Read the model definition and answer for the solid it produces. Units are mm, in the model's axes. A direction names the side the tool comes from. Give positions to 0.01 mm unless a question says otherwise; leave off trailing zeros. Order: outer loops, then holes, each group sorted by start corner. A loop starts at its lowest first (then second) coordinate and runs counter-clockwise, first axis right, second up. Notation, with made-up numbers: (38, 80.5) - (93, 80.5) arc R20 ccw to (93, 107.5) - close; hole circle Ø8 at (-13.5, -37.5). An arc over 180 degrees is marked (long way). Write each question's results on one line, items separated by ' | '.
from build123d import *


with BuildPart() as part:
    # Sketch1 → Revolve1 (revolve)
    with BuildSketch(Plane.XY):
        Polygon((0, 63.5), (0, -63.5), (-31.75, -63.5), (-31.75, 0), (-63.5, 0), (-63.5, 63.5), align=None)
    revolve(axis=Axis((0, 63.5, 0), (0, -1, 0)))

    # Sketch3 → Cut-Revolve1 (revolve, cut)
    with BuildSketch(Plane(origin=(0, 0, 0), x_dir=(0, 0, -1), z_dir=(1, 0, 0))):
        Polygon((-63.5, 44.45), (-31.75, 63.5), (-63.5, 63.5), align=None)
        Polygon((-63.5, 19.05), (-63.5, 0), (-31.75, 0), align=None)
        Polygon((-15.875, -63.5), (-31.75, -50.8), (-31.75, -63.5), align=None)
    revolve(axis=Axis((0, 63.5, 0), (0, -1, 0)), mode=Mode.SUBTRACT)


solid = part.part
(1) For faces 1 (the face through (-29.33, -25.04, 12.16)), 2 (the face through (-60.57, 31.93, -19.07)), determine the directions among +Z, -Z, +X, -X, +Y, -Y from which every point of the face is accessible in a straight line to the end or side of a thin tool.
Conclusion:
face 1: -Y | face 2: +Y, -Y
(2) Section B-B (z = 0) is taken. Give the vertices of the cut face in (x, y) (3 decimals).
Conclusion:
outline: (-63.5, 19.05) - (-31.75, 0) - (-31.75, -50.8) - (-15.875, -63.5) - (15.875, -63.5) - (31.75, -50.8) - (31.75, 0) - (63.5, 19.05) - (63.5, 44.45) - (31.75, 63.5) - (-31.75, 63.5) - (-63.5, 44.45) - close
(3) Section D-D (y = 49.5) is taken. Give the vertices of the cut face in (x, z), plus the area to 3 significant figures.
Conclusion:
outline: circle Ø110.17 at (0, 0) | area: 9,530 mm^2
(4) Consider probe 1 along Z at (x, y) = (-0.5, -0.5); probe 2 along Z at (x, y) = (-12, 28); probe 3 along X at (y, z) = (58, -19.5). Determine where each line is inside the solid, lowest interval first. Write a range as [from, to].
Conclusion:
probe 1: [-31.75, 31.75] | probe 2: [-62.36, 62.36] | probe 3: [-35.97, 35.97]
(5) Each of these flat-tipped pins is pushed along its axis until it touches: pin 1 (1.5 mm diameter, centred on y = -26, z = 34, fed in from +X); pin 2 (8 mm diameter, centred on y = 2.5, z = 20, fed in from -X); pin 3 (1 mm diameter, centred on x = 1.5, y = -43, fed in from +Z); pin 4 (5 mm diameter, centred on x = 20.5, y = -22, fed in from +Z). Where does it stop, or does it pass through?
Conclusion:
pin 1: through | pin 2: x = -37.87 | pin 3: z = 31.73 | pin 4: z = 26.15
(6) Section C-C (y = -10) is taken. Give the vertices of the cut face in (x, z), plus the area to 3 significant figures.
Conclusion:
outline: circle Ø63.5 at (0, 0) | area: 3,170 mm^2
(7) Section A-A (x = 0) is taken. Give the vertices of the cut face in (y, z) (3 decimals).
Conclusion:
outline: (-63.5, -15.875) - (-50.8, -31.75) - (0, -31.75) - (19.05, -63.5) - (44.45, -63.5) - (63.5, -31.75) - (63.5, 31.75) - (44.45, 63.5) - (19.05, 63.5) - (0, 31.75) - (-50.8, 31.75) - (-63.5, 15.875) - close
